from build123d import *

# Parameters (mm, degrees)
SKETCH2_R           = 4.25
BOSS_EXTRUDE1_DEPTH = 6.35
FILLET1_R           = 6


with BuildPart() as part:
    # Sketch2 → Boss-Extrude1 (new body)
    with BuildSketch(Plane.XY):
        with BuildLine():
            Line((11.548494156, -4.783542905), (38.382716246, 60))
            ThreePointArc((38.382716246, 60), (0, 67.634796955), (-38.382716246, 60))
            Line((-38.382716246, 60), (-11.548494156, -4.783542905))
            ThreePointArc((-11.548494156, -4.783542905), (0, -12.5), (11.548494156, -4.783542905))
        make_face()
        with Locations((-27.203312061, 55.222101201)):
            Circle(SKETCH2_R, mode=Mode.SUBTRACT)
        with Locations((-9.56999846, 58.836828221)):
            Circle(SKETCH2_R, mode=Mode.SUBTRACT)
        with Locations((9.56999846, 58.836828221)):
            Circle(SKETCH2_R, mode=Mode.SUBTRACT)
        with Locations((27.203312061, 55.222101201)):
            Circle(SKETCH2_R, mode=Mode.SUBTRACT)
        with Locations((-20.278160914, 38.503307381)):
            Circle(SKETCH2_R, mode=Mode.SUBTRACT)
        with Locations((-7.511195711, 40.953735809)):
            Circle(SKETCH2_R, mode=Mode.SUBTRACT)
        with Locations((7.511195711, 40.953735809)):
            Circle(SKETCH2_R, mode=Mode.SUBTRACT)
        with Locations((20.278160914, 38.503307381)):
            Circle(SKETCH2_R, mode=Mode.SUBTRACT)
        with BuildLine():
            Line((-3.953795645, 3.3), (3.953795645, 3.3))
            ThreePointArc((3.953795645, 3.3), (0, -5.15), (-3.953795645, 3.3))
        make_face(mode=Mode.SUBTRACT)
    extrude(amount=BOSS_EXTRUDE1_DEPTH)

    # Fillet1
    fillet1_edges = [part.edges().sort_by_distance(p)[0] for p in [
        (-38.382716246, 60, 3.175),
        (38.382716246, 60, 3.175),
    ]]
    fillet(fillet1_edges, radius=FILLET1_R)


solid = part.part
The listing builds one solid part. Answer for the finished solid, in the listing's coordinates (mm). A direction names the side the tool comes from. Give positions to 0.01 mm unless a question says otherwise; leave off trailing zeros. Loops run counter-clockwise (first coordinate to the right, second up) from the corner with the lowest first, then second, coordinate; pieces in that order, holes last.
Item 1: Find the intervals of material crossed by line 1 along Y through (x, z) = (-7, 2.5); line 2 along X through (y, z) = (38.5, 2.5); line 3 along Y through (x, z) = (-8, 2), in increasing order.
Derived:
line 1: y = -10.36 to 36.73, 45.17 to 55.45, 62.22 to 67.39
line 2: x = -29.48 to -24.53, -16.03 to -10.98, -4.04 to 4.04, 10.98 to 16.03, 24.53 to 29.48
line 3: y = -9.6 to 36.73, 45.18 to 54.89, 62.79 to 67.32
Item 2: Determine the mould class of faces 3 (the cylindrical face through (0.462, 67.634, 3.131)), 4 (the cylindrical face through (-5.23, 44.54, 3.13)), 5 (the flat face through (-1, 37, 0)) for opening direction Y: +Y half, -Y half, draft (parallel to the pull), parting line (faces both ways), or undercut.
Derived:
face 3: +Y half
face 4: undercut
face 5: draft
Item 3: A cutting plane is placed at A-A (x = 0). Give the vertices of the cut face in (y, z), then the cut area to 3 significant figures.
Derived:
outline: (-12.5, 0) - (-5.15, 0) - (-5.15, 6.35) - (-12.5, 6.35) - close; (3.3, 0) - (67.63, 0) - (67.63, 6.35) - (3.3, 6.35) - close
area: 455 mm2
Item 4: A cutting plane is placed at B-B (y = 52). Give the vertices of the cut face in (x, z).
Derived:
outline: (-35.07, 0) - (-29.97, 0) - (-29.97, 6.35) - (-35.07, 6.35) - close; (-24.43, 0) - (24.43, 0) - (24.43, 6.35) - (-24.43, 6.35) - close; (29.97, 0) - (35.07, 0) - (35.07, 6.35) - (29.97, 6.35) - close
Item 5: A cutting plane is placed at C-C (y = 0). Give the vertices of the cut face in (x, z).
Derived:
outline: (-13.53, 0) - (-5.15, 0) - (-5.15, 6.35) - (-13.53, 6.35) - close; (5.15, 0) - (13.53, 0) - (13.53, 6.35) - (5.15, 6.35) - close
Item 6: Each of these flat-tipped pins is pushed along its axis until it touches: pin 1 Ø1.5 at (x, z) = (18.5, 3) entering from -Y; pin 2 Ø2 at (x, z) = (-20.5, 1.5) entering from -Y; pin 3 Ø1 at (x, z) = (26.5, 4.5) entering from -Y. Where does it stop, or does it pass through?
Derived:
pin 1: stops at y = 10.19
pin 2: stops at y = 14.41
pin 3: stops at y = 30.11
Item 7: A tool of negligible diameter and unlimited length cuts with its end or side. For faces 1 (the flat face through (0, 3.3, 3)), 2 (the cylindrical face through (-0.2, -12.5, 3.1)), from which of +Z, -Z, +X, -X, +Y, -Y can it reach the whole face along a straight path? Write none if from no direction.
Derived:
face 1: +Z, -Z
face 2: +Z, -Z, -Y
Item 8: A cutting plane is placed at D-D (z = 1.75). Give the number of separate pieces and of enclosed holes in the cut face, then the cut area to 3 significant figures.
Derived:
separate pieces: 1
enclosed holes: 9
area: 3,210 mm2
